Can you work these out from the drawing? Everything is in mm from the part's minimum corner. A direction names the side the tool comes from. Round coordinates to 2 decimals unless told otherwise and drop trailing zeros. Write each loop counter-clockwise with the first axis right and the second up, starting at its lowest first coordinate (ties: lowest second). Pieces come first, ordered by that corner, then holes. Notation, with made-up numbers: M 26,73 L 69,73 A20 ccw 69,96 Z; hole C 38.5,36 d5. An arc over 180 degrees is marked long. Use one line per item in the form item = value. Start each with the question number.
Q1. I need wall thicknesses on line 1 along X through (y, z) = (51.5, 4); line 2 along Y through (x, z) = (19, 4.75); line 3 along Y through (x, z) = (17.75, 6.5) (1 decimal). Which ranges of each line are inside material? Lowest first, please. Write a range as from..to.
Q2. I'm going to push flat-ended pins straight in: pin 1 Ø2 at (y, z) = (21, 5.5) entering from -X; pin 2 Ø3 at (x, y) = (13.5, 7) entering from -Z; pin 3 Ø1.2 at (x, y) = (11.5, 10.5) entering from +Z; pin 4 Ø4 at (x, z) = (21.5, 7.5) entering from -Y. Where does each tip first touch, or does it pass through?
Q3. I want a section at C-C on y = 8. List the corners of the cut face in (x, z) for me, and give its area (3 significant figures).
Q4. For the marked faces 1 and 2, which set-ups out of +Z, -Z, +X, -X, +Y, -Y let a thin tool reach every point of the face, with its end or its side?
Q5. I want a section at B-B on z = 2.5. List the corners of the cut face in (x, y) for me, and give its area (3 significant figures).
Q6. I want a section at D-D on z = 19.25. List the corners of the cut face in (x, y) for me, and give its area (3 significant figures).
Q7. I want a section at A-A on z = 10. List the corners of the cut face in (x, y) for me.
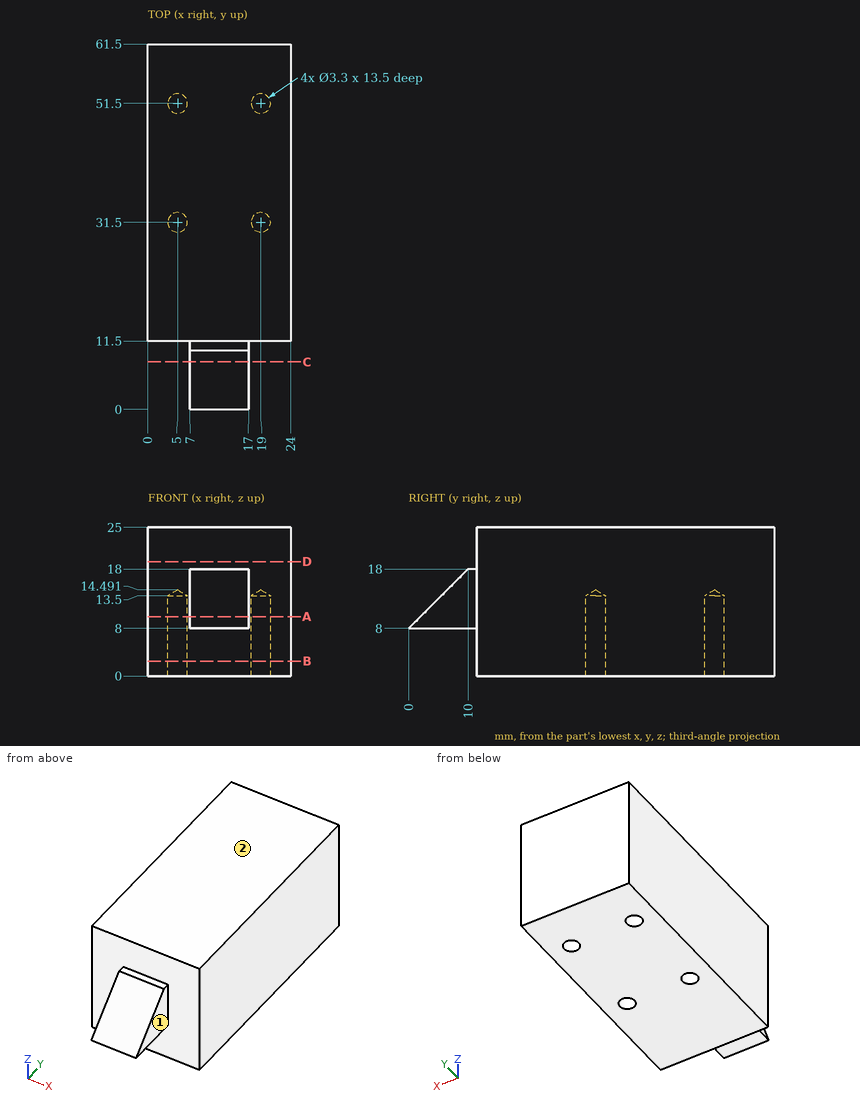
Reported:
q1.line_1 = 0..3.35, 6.65..17.35, 20.65..24
q1.line_2 = 11.5..29.85, 33.15..49.85, 53.15..61.5
q1.line_3 = 11.5..30.4, 32.6..50.4, 52.6..61.5
q2.pin_1 = 0
q2.pin_2 = 8
q2.pin_3 = 18
q2.pin_4 = 11.5
q3.outline = M 7,8 L 17,8 L 17,16 L 7,16 Z
q3.area = 80.0 mm^2
q4.face_1 = +Z, -Z, +X, -Y
q4.face_2 = +Z, +X, -X, +Y, -Y
q5.outline = M 0,11.5 L 24,11.5 L 24,61.5 L 0,61.5 Z; hole C 5,31.5 d3.3; hole C 5,51.5 d3.3; hole C 19,31.5 d3.3; hole C 19,51.5 d3.3
q5.area = 1,170 mm^2
q6.outline = M 0,11.5 L 24,11.5 L 24,61.5 L 0,61.5 Z
q6.area = 1,200 mm^2
q7.outline = M 0,11.5 L 7,11.5 L 7,2 L 17,2 L 17,11.5 L 24,11.5 L 24,61.5 L 0,61.5 Z; hole C 5,31.5 d3.3; hole C 5,51.5 d3.3; hole C 19,31.5 d3.3; hole C 19,51.5 d3.3
